Input: part model. Units: mm. Frame: model coordinates. Round coordinates to 2 decimals unless told otherwise and drop trailing zeros. Loops run counter-clockwise (first coordinate to the right, second up) from the corner with the lowest first, then second, coordinate; pieces in that order, holes last.
(1) First-contact query: pin 1 Ø3 at (y, z) = (-3, 0.5) entering from -X; pin 2 Ø1 at (x, y) = (-8, -5.5) entering from +Z; pin 3 Ø2 at (x, y) = (-23, -1) entering from -Z. Flat tips, straight axial feed; report the tip coordinate or a pass-through.
(2) Cut plane B-B, the plane z = 18. Output: boundary loops of the cut face in (x, y).
(3) Cut plane A-A, the plane x = 22. Output: boundary loops of the cut face in (y, z), and give its area (3 significant figures).
(4) Line query: line 1 (X direction, y = -3.5, z = -33); line 2 (X direction, y = -2, z = -15.5). Output: solid intervals per line, ascending.
from build123d import *

# Parameters (mm, degrees)
F0_W     = 76.2
F0_H     = 76.2
F1_DEPTH = 6.35
F2_W     = 6.35
F2_H     = 6.35
F3_DEPTH = 6.351
F4_W     = 6.35
F4_H     = 6.35
F5_DEPTH = 6.351
F6_W     = 6.35
F6_H     = 6.35
F6_H_2   = 12.7
F7_DEPTH = 6.351


# Not quite as in the source:
# - a feature names something its author has since deleted; it is built from what else it names


with BuildPart() as f1:
    # F0 (on Front) → F1 (new body)
    with BuildSketch(Plane.XZ):
        Rectangle(F0_W, F0_H)
    extrude(amount=F1_DEPTH)

    # F2 (on face) → F3 (cut, through all)
    with BuildSketch(Plane.XZ.offset(6.35)):
        with Locations((-22.225, 34.925)):
            Rectangle(F2_W, F2_H)
        with Locations((-9.525, 34.925)):
            Rectangle(F2_W, F2_H)
        with Locations((9.525, 34.925)):
            Rectangle(F2_W, F2_H)
        with Locations((22.225, 34.925)):
            Rectangle(F2_W, F2_H)
    extrude(amount=-F3_DEPTH, mode=Mode.SUBTRACT)

    # F4 (on face) → F5 (cut, through all)
    with BuildSketch(Plane.XZ.offset(6.35)):
        with Locations((-9.525, -34.925)):
            Rectangle(F4_W, F4_H)
        with Locations((9.525, -34.925)):
            Rectangle(F4_W, F4_H)
        with Locations((22.225, -34.925)):
            Rectangle(F4_W, F4_H)
        with Locations((-22.225, -34.925)):
            Rectangle(F4_W, F4_H)
    extrude(amount=-F5_DEPTH, mode=Mode.SUBTRACT)

    # F6 (on face) → F7 (cut, through all)
    with BuildSketch(Plane.XZ.offset(6.35)):
        with Locations((-34.925, -28.575)):
            Rectangle(F6_W, F6_H)
        with Locations((-34.925, -15.875)):
            Rectangle(F6_W, F6_H)
        with Locations((-34.925, 0)):
            Rectangle(F6_W, F6_H_2)
        with Locations((-34.925, 15.875)):
            Rectangle(F6_W, F6_H)
        with Locations((-34.925, 28.575)):
            Rectangle(F6_W, F6_H)
        with Locations((34.925, -28.575)):
            Rectangle(F6_W, F6_H)
        with Locations((34.925, -15.875)):
            Rectangle(F6_W, F6_H)
        with Locations((34.925, -3.175)):
            Rectangle(F6_W, F6_H)
        with Locations((34.925, 3.175)):
            Rectangle(F6_W, F6_H)
        with Locations((34.925, 15.875)):
            Rectangle(F6_W, F6_H)
        with Locations((34.925, 28.575)):
            Rectangle(F6_W, F6_H)
    extrude(amount=-F7_DEPTH, mode=Mode.SUBTRACT)


solid = f1.part
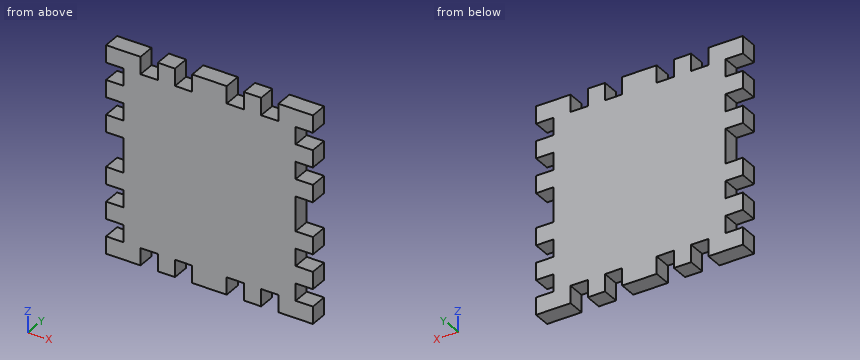
Reported:
1. pin 1: stops at x = -31.75
1. pin 2: stops at z = 31.75
1. pin 3: stops at z = -31.75
2. outline: (-31.75, -6.35) - (31.75, -6.35) - (31.75, 0) - (-31.75, 0) - close
3. outline: (-6.35, -31.75) - (0, -31.75) - (0, 31.75) - (-6.35, 31.75) - close
3. area: 403 mm2
4. line 1: x = -38.1 to -25.4, -19.05 to -12.7, -6.35 to 6.35, 12.7 to 19.05, 25.4 to 38.1
4. line 2: x = -31.75 to 31.75
